Can you work these out from the model? Positions are in its coordinate system, mm. Face numbers are marked on the shaded views. A direction names the side the tool comes from. Round coordinates to 2 decimals unless told otherwise and drop trailing zeros. Order: outer loops, then holes, each group sorted by start corner. A loop starts at its lowest first (then second) coordinate and runs counter-clockwise, first axis right, second up. Notation, with made-up numbers: (55.5, -4) -> (93.5, -4) arc R14 ccw to (93.5, 11) -> close; hole circle Ø1 at (18.25, 18). An arc over 180 degrees is marked (long way). One line per item, written item: value.
```python
from build123d import *

# Parameters (mm, degrees)
SKETCH1_R           = 11.5
SKETCH1_R_2         = 1.5
BOSS_EXTRUDE1_DEPTH = 1.5
SKETCH2_W           = 1.5
SKETCH2_H           = 1.5
BOSS_EXTRUDE3_DEPTH = 3.5
SKETCH3_W           = 1.5
SKETCH3_H           = 1.5
BOSS_EXTRUDE4_DEPTH = 1
CHAMFER2_SIZE       = 2
CHAMFER2_SIZE2      = 0.932615316
SKETCH5_W           = 1.5
SKETCH5_H           = 1.5
BOSS_EXTRUDE6_DEPTH = 1
CHAMFER5_SIZE       = 2
CHAMFER5_SIZE2      = 0.932615316


with BuildPart() as part:
    # Sketch1 → Boss-Extrude1 (new body)
    with BuildSketch(Plane.XY):
        Circle(SKETCH1_R)
        Circle(SKETCH1_R_2, mode=Mode.SUBTRACT)
    extrude(amount=BOSS_EXTRUDE1_DEPTH)

    # Sketch2 → Boss-Extrude3 (add)
    with BuildSketch(Plane.XY.offset(1.5)):
        with Locations((4.948341792, 3.393215807)):
            Rectangle(SKETCH2_W, SKETCH2_H)
        with Locations((-4.948341792, -3.393215807)):
            Rectangle(SKETCH2_W, SKETCH2_H)
    extrude(amount=BOSS_EXTRUDE3_DEPTH)

    # Sketch3 → Boss-Extrude4 (add)
    with BuildSketch(Plane(origin=(0, 4.143215807, 0), x_dir=(1, 0, 0), z_dir=(0, 1, 0))):
        with Locations((4.948341792, -4.25)):
            Rectangle(SKETCH3_W, SKETCH3_H)
    extrude(amount=BOSS_EXTRUDE4_DEPTH)

    # Chamfer2
    chamfer2_edges = [part.edges().sort_by_distance(p)[0] for p in [
        (5.698341792, 5.143215807, 4.25),
    ]]
    chamfer2_side = [part.faces().sort_by_distance(p)[0] for p in [
        (5.698341792, 3.670993585, 3.472222222),
    ]]
    chamfer(chamfer2_edges, length=CHAMFER2_SIZE, length2=CHAMFER2_SIZE2, reference=chamfer2_side[0])

    # Sketch5 → Boss-Extrude6 (add)
    with BuildSketch(Plane.XZ.offset(4.143215807)):
        with Locations((-4.948341792, 4.25)):
            Rectangle(SKETCH5_W, SKETCH5_H)
    extrude(amount=BOSS_EXTRUDE6_DEPTH)

    # Chamfer5
    chamfer5_edges = [part.edges().sort_by_distance(p)[0] for p in [
        (-5.698341792, -5.143215807, 4.25),
    ]]
    chamfer5_side = [part.faces().sort_by_distance(p)[0] for p in [
        (-5.698341792, -3.670993585, 3.472222222),
    ]]
    chamfer(chamfer5_edges, length=CHAMFER5_SIZE, length2=CHAMFER5_SIZE2, reference=chamfer5_side[0])


solid = part.part
```
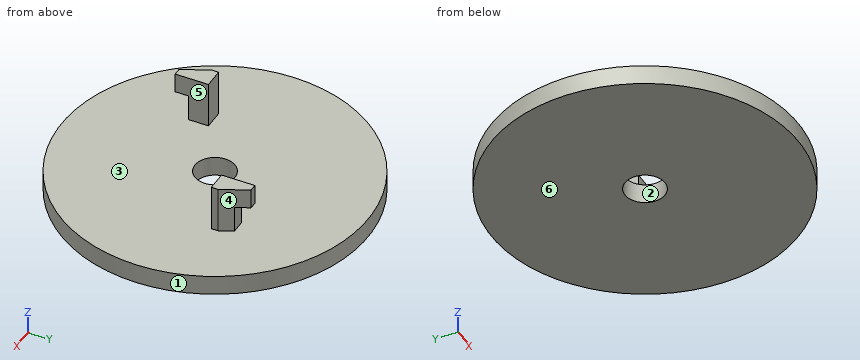
Q1. I want a section at D-D on z = 3.8. List the corners of the cut face in (x, y) for me, plus the area to 3 significant figures.
Answers below:
outline: (-5.7, -3.14) -> (-4.77, -5.14) -> (-4.2, -5.14) -> (-4.2, -2.64) -> (-5.7, -2.64) -> close; (4.2, 2.64) -> (5.7, 2.64) -> (5.7, 3.14) -> (4.77, 5.14) -> (4.2, 5.14) -> close
area: 5.63 mm^2
Q2. Please list where these lines run through material, in increasing order: line 1 along Y through (x, z) = (0, 0.35); line 2 along Z through (x, y) = (-5, -0.25); line 3 along Y through (x, z) = (-4.25, 4.75).
Answers below:
line 1: -11.5 to -1.5, 1.5 to 11.5
line 2: 0 to 1.5
line 3: -5.14 to -2.64
Q3. I want a section at B-B on x = 0. List the corners of the cut face in (y, z) for me.
Answers below:
outline: (-11.5, 0) -> (-1.5, 0) -> (-1.5, 1.5) -> (-11.5, 1.5) -> close; (1.5, 0) -> (11.5, 0) -> (11.5, 1.5) -> (1.5, 1.5) -> close
Q4. We'd pull the mould along Y, two halves only. Please class the marked faces 1, 2 and 3: released by +Y, released by -Y, zero draft, split by the parting line, or undercut.
Answers below:
face 1: split by the parting line
face 2: undercut
face 3: zero draft
Q5. On a 3-axis mill with a long thin cutter (end or side, diameter ignored), from which of +Z, -Z, +X, -X, +Y, -Y can I reach the whole of each face in a straight line? I mean the marked faces 4, 5 and 6. Say none if no direction works.
Answers below:
face 4: +Z, +X, +Y
face 5: +Z, +X, +Y, -Y
face 6: -Z, +X, -X, +Y, -Y
Q6. I want a section at A-A on z = 2.4. List the corners of the cut face in (x, y) for me, plus the area to 3 significant figures.
Answers below:
outline: (-5.7, -3.14) -> (-5.23, -4.14) -> (-4.2, -4.14) -> (-4.2, -2.64) -> (-5.7, -2.64) -> close; (4.2, 2.64) -> (5.7, 2.64) -> (5.7, 3.14) -> (5.23, 4.14) -> (4.2, 4.14) -> close
area: 4.03 mm^2
Q7. Will these pins go through, and if not, where does the flat tip stop? pin 1 Ø12 at (x, y) = (2, -7) entering from +Z; pin 2 Ø0.8 at (y, z) = (4, 4) entering from -X; pin 3 Ø0.8 at (x, z) = (-4.5, 3) entering from -Y; pin 4 Ø1.5 at (y, z) = (-1.5, 3) entering from -X.
Answers below:
pin 1: z = 1.5
pin 2: x = 4.2
pin 3: y = -4.14
pin 4: through
